Could you check a few things on this model? Use its own coordinates, in mm. Face numbers are marked on the shaded views. A direction names the side the tool comes from. Coordinates: 2 decimals unless noted, no trailing zeros. Order: outer loops, then holes, each group sorted by start corner. A loop starts at its lowest first (then second) coordinate and runs counter-clockwise, first axis right, second up. Notation, with made-up numbers: M -34.75,34 L -29.75,34 A16 ccw -29.75,55 Z; hole C 23.5,67 d9. An arc over 180 degrees is marked long. One line per question, with ' | ' between items. Start each with the question number.
from build123d import *

# Parameters (mm, degrees)
SKETCH_1_R          = 2
EXTRUDE_1_DEPTH     = 5
SKETCH_2_W          = 105.590665855
SKETCH_2_H          = 53.734325109
CUT_EXTRUDE_1_DEPTH = 2
SKETCH_4_R          = 1.5
CUT_EXTRUDE_2_DEPTH = 3


with BuildPart() as part:
    # 草图1 → 凸台-拉伸1 (new body)
    with BuildSketch(Plane.XY):
        with BuildLine():
            Line((-10.191413347, 2.526874351), (-19, -33))
            Line((-19, -33), (-19, -34))
            Line((-19, -34), (33, -34))
            Line((33, -34), (33, -33))
            Line((33, -33), (8.904718959, 5.563809869))
            ThreePointArc((8.904718959, 5.563809869), (-1.649133089, 10.369684665), (-10.191413347, 2.526874351))
        make_face()
        Circle(SKETCH_1_R, mode=Mode.SUBTRACT)
        with BuildLine():
            Line((-8.452697078, -7.081843943), (-13.519839571, -27.5186906))
            ThreePointArc((-13.519839571, -27.5186906), (-13.153835237, -29.232351654), (-11.578617982, -30))
            Line((-11.578617982, -30), (22.801020138, -30))
            ThreePointArc((22.801020138, -30), (24.55024091, -28.969652872), (24.497157083, -26.940226692))
            Line((24.497157083, -26.940226692), (9.642502803, -3.165776319))
            ThreePointArc((9.642502803, -3.165776319), (7.876643723, -2.22676529), (6.180506778, -3.286538599))
            ThreePointArc((6.180506778, -3.286538599), (1.099422059, -6.91312311), (-4.856029369, -5.041723789))
            ThreePointArc((-4.856029369, -5.041723789), (-6.797250959, -4.560414389), (-8.184687922, -6.0009069))
            Line((-8.184687922, -6.0009069), (-8.452697078, -7.081843943))
        make_face(mode=Mode.SUBTRACT)
    extrude(amount=EXTRUDE_1_DEPTH)

    # 草图2 → 切除-拉伸1 (cut)
    with BuildSketch(Plane.XY.offset(5)):
        with Locations((1.500851151, -4.132837446)):
            Rectangle(SKETCH_2_W, SKETCH_2_H)
    extrude(amount=-CUT_EXTRUDE_1_DEPTH, mode=Mode.SUBTRACT)

    # 草图4 → 切除-拉伸2 (cut)
    with BuildSketch(Plane(origin=(0, -34, 0), x_dir=(-1, 0, 0), z_dir=(0, -1, 0))):
        with Locations(Location((14, -2.5, 0), (0, 0, 90))):
            Circle(SKETCH_4_R)
        with Locations(Location((-28, -2.5, 0), (0, 0, 90))):
            Circle(SKETCH_4_R)
    extrude(amount=-CUT_EXTRUDE_2_DEPTH, mode=Mode.SUBTRACT)


solid = part.part
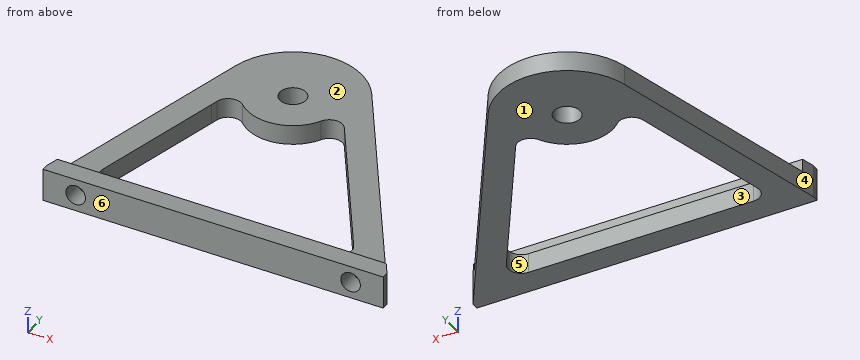
(1) Imagine slicing it at A-A, the plane x = 0. Write out the boundary of the cut face in (y, z), plus the area to 3 significant figures.
(2) Imagine slicing it at B-B, the plane y = -28.5. Write out the boundary of the cut face in (x, z), plus the area to 3 significant figures.
(3) If I drill on line 1 along Y through (x, z) = (0, 2.05); line 2 along Z through (x, y) = (-14, -32); line 3 along X through (y, z) = (-32, 2.5), over which ranges is the centre line in solid material (lowest first)? Write a range as from..to.
(4) Imagine slicing it at C-C, the plane x = 22. Write out the boundary of the cut face in (y, z), plus the area to 3 significant figures.
(5) We'd pull the mould along X, two halves only. Please class the marked faces 4, 5 and 6: +X half, -X half, draft (parallel to the pull), parting line (faces both ways), or undercut.
(6) Imagine slicing it at D-D, the plane x = 28. Write out the boundary of the cut face in (y, z).
(7) For P1, Ø2.5, axis at x = 0, y = 0, coming from the -Z side; P2, Ø2.5, axis at x = 12.5, z = 1, coming from the +Y side; P3, Ø1.5, axis at x = 15.5, y = -11.5, coming from the +Z side, each with a flat end and sliding along its axis, tell me the tip position at first contact or that it passes through.
(8) On a 3-axis mill with a long thin cutter (end or side, diameter ignored), from which of +Z, -Z, +X, -X, +Y, -Y can I reach the whole of each face in a straight line? I mean the marked faces 1, 2 and 3. Say none if no direction works.
Answers:
1) outline: M -34,0 L -30,0 L -30,3 L -31,3 L -31,5 L -34,5 Z; M -7,0 L -2,0 L -2,3 L -7,3 Z; M 2,0 L 10.5,0 L 10.5,3 L 2,3 Z | area: 58.5 mm²
2) outline: M -17.88,0 L -13.52,0 L -13.52,3 L -17.88,3 Z; M 24.74,0 L 30.19,0 L 30.19,3 L 24.74,3 Z | area: 29.5 mm²
3) line 1: -34..-30, -7..-2, 2..10.5 | line 2: 0..1, 4..5 | line 3: -18.75..-15.5, -12.5..26.5, 29.5..32.38
4) outline: M -34,0 L -30,0 L -30,3 L -31,3 L -31,5 L -34,5 Z; M -22.94,0 L -15.39,0 L -15.39,3 L -22.94,3 Z | area: 40.6 mm²
5) face 4: -X half | face 5: undercut | face 6: draft
6) outline: M -34,0 L -25,0 L -25,3 L -31,3 L -31,1 L -34,1 Z; M -34,4 L -31,4 L -31,5 L -34,5 Z
7) P1: through | P2: y = 1.81 | P3: z = 3
8) face 1: -Z, +X, -X, +Y, -Y | face 2: +Z, +X, -X, +Y | face 3: +Z, -Z
